Here's how the part is built. I have some questions about the finished solid (model axes, mm). Face numbers are marked on the shaded views. A direction names the side the tool comes from. Give positions to 0.01 mm unless a question says otherwise; leave off trailing zeros. Write each loop counter-clockwise with the first axis right and the second up, starting at its lowest first coordinate (ties: lowest second). Pieces come first, ordered by that corner, then holes. Notation, with made-up numbers: M 7.25,-13.75 L 44.25,-13.75 A25 ccw 44.25,1.25 Z; hole C -24.75,-3 d7. An arc over 180 degrees is marked long. Answer as CSV lines item,"result". Start each with the question number.
Q1. For pin 1 (4 mm diameter, centred on x = 1, z = -7.5, fed in from -Y); pin 2 (2 mm diameter, centred on y = 1, z = -3.5, fed in from +X); pin 3 (4 mm diameter, centred on x = 0.5, y = 3, fed in from -Z), each with a flat end and sliding along its axis, tell me the tip position at first contact or that it passes through.
Q2. If I drill on line 1 along Z through (x, y) = (-2.5, -1.75); line 2 along X through (y, z) = (0, -10.5); line 3 along Y through (x, z) = (1.25, -14.75), over which ranges is the centre line in solid material (lowest first)?
Q3. Suppose I cut it at C-C (z = -6.75). Write out the boundary of the cut face in (x, y), then the cut area to 3 significant figures.
Q4. Suppose I cut it at D-D (z = 0.5). Write out the boundary of the cut face in (x, y), then the cut area to 3 significant figures.
Q5. On a 3-axis mill with a long thin cutter (end or side, diameter ignored), from which of +Z, -Z, +X, -X, +Y, -Y can I reach the whole of each face in a straight line? I mean the marked faces 1 and 2. Say none if no direction works.
```python
from build123d import *

# Parameters (mm, degrees)
F0_R     = 4.0005
F0_R_2   = 2.9972
F1_DEPTH = 2.0066
F2_SIZE  = 0.762
F3_DEPTH = 8.001
F5_SIZE  = 0.762
F4_R     = 2.261837
F6_DEPTH = 10.0076
F7_SIZE  = 0.762


with BuildPart() as f1:
    # F0 (on Top) → F1 (new body)
    with BuildSketch(Plane.XY):
        Circle(F0_R)
        Circle(F0_R_2, mode=Mode.SUBTRACT)
        Circle(F0_R_2)
    extrude(amount=F1_DEPTH)

    # F2
    f2_edges = [f1.edges().sort_by_distance(p)[0] for p in [
        (-4.0005, 0, 2.0066),
    ]]
    chamfer(f2_edges, length=F2_SIZE)

    # F0 (on Top) → F3 (join)
    with BuildSketch(Plane.XY):
        Circle(F0_R_2)
    extrude(amount=-F3_DEPTH)

    # F5
    f5_edges = [f1.edges().sort_by_distance(p)[0] for p in [
        (-2.9972, 0, -8.001),
    ]]
    chamfer(f5_edges, length=F5_SIZE)

    # F4 (on face) → F6 (join)
    with BuildSketch(Plane(origin=(0, 0, -8.001), x_dir=(1, 0, 0), z_dir=(0, 0, -1))):
        Circle(F4_R)
    extrude(amount=F6_DEPTH)

    # F7
    f7_edges = [f1.edges().sort_by_distance(p)[0] for p in [
        (-2.261837, 0, -18.0086),
    ]]
    chamfer(f7_edges, length=F7_SIZE)


solid = f1.part
```
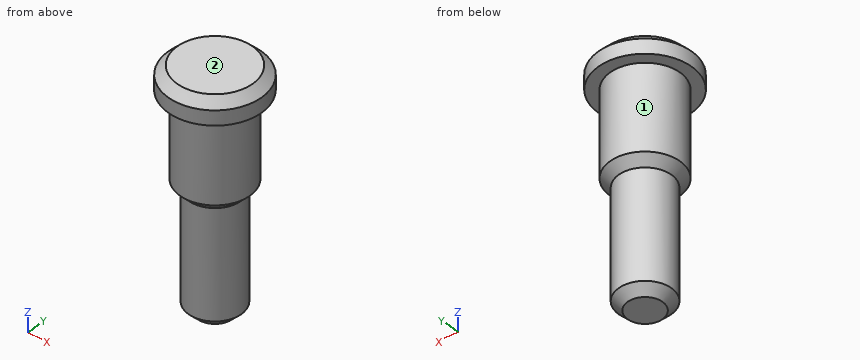
Resolved:
1,pin 1,"y = -3"
1,pin 2,"x = 3"
1,pin 3,"z = -18.01"
2,line 1,"0 to 2.01"
2,line 2,"-2.26 to 2.26"
2,line 3,"-1.89 to 1.89"
3,outline,"C 0,0 d5.99"
3,area,"28.2 mm^2"
4,outline,"C 0,0 d8"
4,area,"50.3 mm^2"
5,face 1,"-Z"
5,face 2,"+Z, +X, -X, +Y, -Y"
